```python
from build123d import *

# Parameters (mm, degrees)
SKETCH1_R           = 19.05
BOSS_EXTRUDE1_DEPTH = 25.4
SKETCH2_W           = 101.6
SKETCH2_H           = 25.4
BOSS_EXTRUDE2_DEPTH = 57.15
SKETCH5_W           = 101.6
SKETCH5_H           = 25.4
BOSS_EXTRUDE3_DEPTH = 88.9
SKETCH6_R           = 50.8
BOSS_EXTRUDE4_DEPTH = 50.8
SKETCH7_R           = 25.4
CUT_EXTRUDE1_DEPTH  = 50.8
FILLET1_R           = 12.7
FILLET2_R           = 38.1


with BuildPart() as part:
    # Sketch1 → Boss-Extrude1 (new body)
    with BuildSketch(Plane.XY):
        with BuildLine():
            Line((-88.9, 38.1), (88.9, 38.1))
            ThreePointArc((88.9, 38.1), (127, 0), (88.9, -38.1))
            Line((88.9, -38.1), (-88.9, -38.1))
            ThreePointArc((-88.9, -38.1), (-127, 0), (-88.9, 38.1))
        make_face()
        with Locations((-88.9, 0)):
            Circle(SKETCH1_R, mode=Mode.SUBTRACT)
        with Locations((88.9, 0)):
            Circle(SKETCH1_R, mode=Mode.SUBTRACT)
    extrude(amount=-BOSS_EXTRUDE1_DEPTH)

    # Sketch2 → Boss-Extrude2 (add)
    with BuildSketch(Plane(origin=(0, 0, -25.4), x_dir=(-1, 0, 0), z_dir=(0, 0, -1))):
        with Locations((0, 25.4)):
            Rectangle(SKETCH2_W, SKETCH2_H)
    extrude(amount=BOSS_EXTRUDE2_DEPTH)

    # Sketch5 → Boss-Extrude3 (add)
    with BuildSketch(Plane(origin=(0, 38.1, 0), x_dir=(1, 0, 0), z_dir=(0, 1, 0))):
        with Locations((0, 69.85)):
            Rectangle(SKETCH5_W, SKETCH5_H)
    extrude(amount=BOSS_EXTRUDE3_DEPTH)

    # Sketch6 → Boss-Extrude4 (add)
    with BuildSketch(Plane.XY.offset(-57.15)):
        with Locations((0, 127)):
            Circle(SKETCH6_R)
    extrude(amount=-BOSS_EXTRUDE4_DEPTH)

    # Sketch7 → Cut-Extrude1 (cut)
    with BuildSketch(Plane.XY.offset(-57.15)):
        with Locations((0, 127)):
            Circle(SKETCH7_R)
    extrude(amount=-CUT_EXTRUDE1_DEPTH, mode=Mode.SUBTRACT)

    # Fillet1
    fillet1_edges = [part.edges().sort_by_distance(p)[0] for p in [
        (0, 38.1, -57.15),
    ]]
    fillet(fillet1_edges, radius=FILLET1_R)

    # Fillet2
    fillet2_edges = [part.edges().sort_by_distance(p)[0] for p in [
        (0, 12.7, -82.55),
    ]]
    fillet(fillet2_edges, radius=FILLET2_R)


solid = part.part
```
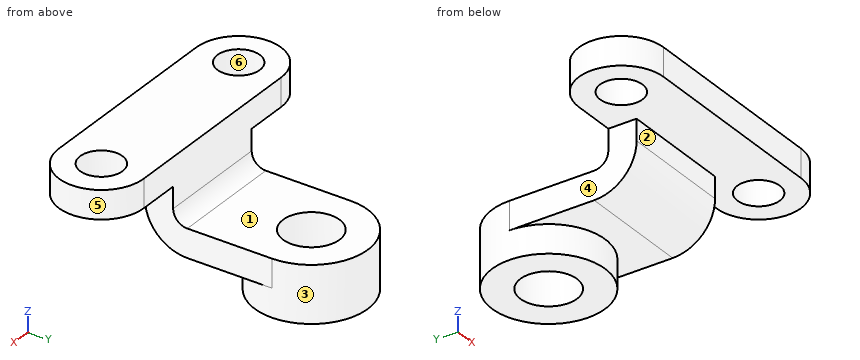
Read the model definition and answer for the solid it produces. Units are mm, in the model's axes. Face numbers are marked on the shaded views. A direction names the side the tool comes from. Coordinates: 2 decimals unless noted, no trailing zeros. Loops run counter-clockwise (first coordinate to the right, second up) from the corner with the lowest first, then second, coordinate; pieces in that order, holes last. Notation, with made-up numbers: (-3, 52.5) -> (32, 52.5) arc R13 ccw to (32, 56.5) -> close; hole circle Ø5 at (69.25, -37.5). An arc over 180 degrees is marked (long way). Return JSON: item names as keys, results as strings.
Item 1: Flat-ended cylindrical pins translate along their axes: P1, Ø17, axis at y = 66.5, z = -61, coming from the +X side; P2, Ø10, axis at x = -13.5, z = -37, coming from the +Y side; P3, Ø4, axis at y = 91, z = -85.5, coming from the -X side; P4, Ø3, axis at y = 22, z = -74, coming from the +X side. Find the tip coordinate at first contact, or state that the pin passes through.
Answers:
{"P1": "stops at x = 50.8", "P2": "stops at y = 38.1", "P3": "stops at x = -37.74", "P4": "passes through"}
Item 2: Find section C-C (y = 119.5). Determine the outline of the cut face in (x, z).
Answers:
{"outline": "(-50.8, -82.55) -> (-50.24, -82.55) -> (-50.24, -107.95) -> (-24.27, -107.95) -> (-24.27, -57.15) -> (-50.8, -57.15) -> close; (24.27, -107.95) -> (50.24, -107.95) -> (50.24, -82.55) -> (50.8, -82.55) -> (50.8, -57.15) -> (24.27, -57.15) -> close"}
Item 3: Find section B-B (y = 0). Determine the outline of the cut face in (x, z), plus the area to 3 significant figures.
Answers:
{"outline": "(-127, -25.4) -> (-107.95, -25.4) -> (-107.95, 0) -> (-127, 0) -> close; (-69.85, -25.4) -> (69.85, -25.4) -> (69.85, 0) -> (-69.85, 0) -> close; (107.95, -25.4) -> (127, -25.4) -> (127, 0) -> (107.95, 0) -> close", "area": "4,520 mm2"}
Item 4: For the marked faces 1, 2 and 3, determine the directions among +Z, -Z, +X, -X, +Y, -Y from which every point of the face is accessible in a straight line to the end or side of a thin tool.
Answers:
{"face 1": "+Z, +X, -X, +Y", "face 2": "-Z, +X, -X, -Y", "face 3": "-Z"}
Item 5: Find section A-A (x = 0). Determine the outline of the cut face in (y, z).
Answers:
{"outline": "(-38.1, -25.4) -> (12.7, -25.4) -> (12.7, -44.45) arc R38.1 ccw to (50.8, -82.55) -> (76.2, -82.55) -> (76.2, -107.95) -> (101.6, -107.95) -> (101.6, -57.15) -> (50.8, -57.15) arc R12.7 cw to (38.1, -44.45) -> (38.1, 0) -> (-38.1, 0) -> close; (152.4, -107.95) -> (177.8, -107.95) -> (177.8, -57.15) -> (152.4, -57.15) -> close"}
Item 6: Find the intervals of material crossed by probe 1 along Y at (x, z) = (0, -93); probe 2 along Y at (x, z) = (-88.9, -9); probe 3 along Z at (x, y) = (33.5, 11), in increasing order.
Answers:
{"probe 1": "y = 76.2 to 101.6, 152.4 to 177.8", "probe 2": "y = -38.1 to -19.05, 19.05 to 38.1", "probe 3": "z = -25.4 to 0"}
Item 7: For a pull along X with two mould halves and no side action, classify the marked faces 4, 5 and 6 as +X half, -X half, draft (parallel to the pull), parting line (faces both ways), or undercut.
Answers:
{"face 4": "-X half", "face 5": "+X half", "face 6": "undercut"}
Item 8: Find section D-D (z = -71). Determine the outline of the cut face in (x, y), plus the area to 3 significant figures.
Answers:
{"outline": "(-50.8, 23.47) -> (50.8, 23.47) -> (50.8, 127) arc R50.8 ccw to (-50.8, 127) -> close; hole circle Ø50.8 at (0, 127)", "area": "12,500 mm2"}
